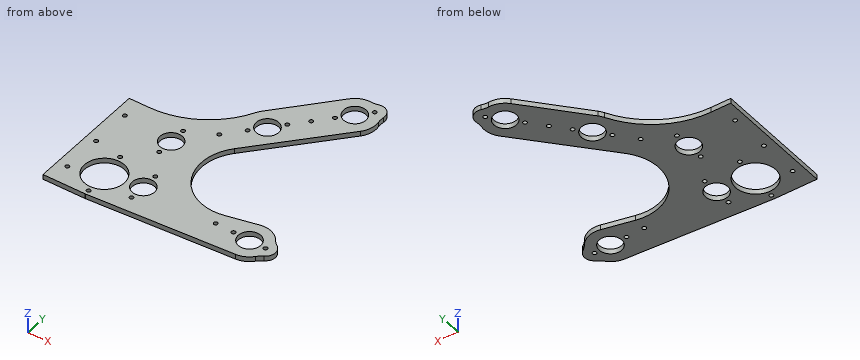
Autodesk Inventor part; units mm, degrees
ref_plane "YZ Plane" through (0, 0, 0) normal (1, 0, 0) x (0, 1, 0)
ref_plane "XZ Plane" through (0, 0, 0) normal (0, 1, 0) x (-1, 0, 0)
ref_plane "XY Plane" through (0, 0, 0) normal (0, 0, 1) x (1, 0, 0)
sketch "Sketch1" plane through (0, 0, 0) normal (0, 0, 1) x (1, 0, 0)
  line L0 (0, 0) -> (704.681, 0) construction
  line L1 (704.681, 0) -> (704.681, 101.6) construction
  line L2 (704.681, 101.6) -> (0, 101.6) construction
  circle A0 centre (304.8, 38.1) radius 38.1 construction
  circle A1 centre (212.725, 197.5786) radius 38.1 construction
  circle A2 centre (274.2046, 266.7) radius 38.1 construction
  circle A3 centre (499.5893, 180.5177) radius 203.2 construction
  line L3 (78.3329, 304.8) -> (550.894, 304.8) construction
  circle A4 centre (247.764, 111.4893) radius 57.15 construction
  circle A5 centre (258.7625, 117.8393) radius 53.975 construction
  line L4 (212.725, 197.5786) -> (304.8, 38.1) construction
  line L5 (258.7625, 117.8393) -> (247.764, 111.4893) construction
  line L6 (274.2046, 266.7) -> (212.725, 197.5786) construction
  dimension "d0" = 101.6
  dimension "d2" = 76.2
  dimension "d3" = 76.2
  dimension "d4" = 76.2
  dimension "d8" = 406.4
  dimension "d9" = 304.8
  dimension "d11" = 304.8
  dimension "d13" = 114.3
  dimension "d14" = 107.95
  dimension "d15" = 12.7
  dimension "d16" = 92.5068
  dimension "d17" = 60
sketch "Sketch4" plane through (0, 0, 0) normal (0, 0, 1) x (1, 0, 0)
  circle A0 centre (274.2046, 266.7) radius 38.1 construction
  circle A1 centre (212.725, 197.5786) radius 38.1 construction
  circle A2 centre (247.764, 111.4893) radius 57.15 construction
  circle A3 centre (304.8, 38.1) radius 38.1 construction
  circle A4 centre (274.2046, 266.7) radius 14.2875
  circle A5 centre (212.725, 197.5786) radius 14.2875
  circle A6 centre (304.8, 38.1) radius 14.2875
  circle A7 centre (145.2547, 121.0056) radius 39.6875 construction
  circle A8 centre (165.2583, 44.1925) radius 39.6875 construction
  circle A9 centre (145.2547, 121.0056) radius 14.2875
  circle A10 centre (165.2583, 44.1925) radius 14.2875
  line L0 (304.8, 38.1) -> (165.2583, 44.1925) construction
  line L1 (145.2547, 121.0056) -> (212.725, 197.5786) construction
  circle A11 centre (165.2583, 44.1925) radius 23.876 construction
  circle A12 centre (145.2547, 121.0056) radius 23.876 construction
  line L2 (128.9029, 138.4033) -> (202.94, 207.9895) construction
  line L3 (164.5725, 106.974) -> (224.2849, 189.182) construction
  line L4 (165.8568, 20.324) -> (305.1581, 23.817) construction
  line L5 (306.4016, 52.2974) -> (167.9348, 67.918) construction
  circle A13 centre (120.0426, 37.9792) radius 5.9531 construction
  circle A14 centre (120.0426, 37.9792) radius 25.4
  circle A15 centre (117.2754, 69.6084) radius 6.35 construction
  circle A16 centre (122.8098, 6.35) radius 6.35 construction
  line L6 (117.2754, 69.6084) -> (122.8098, 6.35) construction
  line L7 (0, 0) -> (304.8, 0) construction
  line L8 (69.2426, 0) -> (94.6426, 0) construction
  line L9 (94.6426, 0) -> (94.6426, 152.4) construction
  line L10 (94.6426, 152.4) -> (69.2426, 152.4)
  line L11 (69.2426, 152.4) -> (69.2426, 0)
  line L12 (81.9426, 127) -> (81.9426, 25.4) construction
  line L13 (283.8015, 39.0168) -> (325.7985, 37.1832) construction
  line L14 (260.2358, 250.9949) -> (288.1734, 282.4051) construction
  line L15 (145.2547, 99.9871) -> (145.2547, 142.0241) construction
  line L16 (165.2583, 23.174) -> (165.2583, 65.211) construction
  line L17 (226.6204, 213.3487) -> (198.8296, 181.8085) construction
  circle A17 centre (304.8, 38.1) radius 26.9875 construction
  circle A18 centre (325.7985, 37.1832) radius 12.7 construction
  circle A19 centre (288.1734, 282.4051) radius 12.7 construction
  line L18 (274.2046, 266.7) -> (212.725, 197.5786) construction
  circle A20 centre (274.2046, 266.7) radius 26.9875 construction
  circle A21 centre (212.725, 197.5786) radius 26.9875 construction
  arc A22 (94.6426, 152.4) -> (188.7085, 209.8884) centre (94.6426, 258.1022) ccw
  line L19 (254.0394, 284.6358) -> (192.5598, 215.5143)
  arc A23 (280.9291, 292.8363) -> (254.0394, 284.6358) centre (274.2046, 266.7) ccw
  arc A24 (299.3783, 276.4268) -> (280.9291, 292.8363) centre (288.1734, 282.4051) ccw
  line L20 (205.2733, 149.7079) -> (294.2696, 248.6523)
  arc A25 (205.2733, 149.7079) -> (260.3346, 55.7389) centre (247.764, 111.4893) ccw
  line L21 (260.3346, 55.7389) -> (298.8639, 64.4266)
  arc A26 (294.2696, 248.6523) -> (299.3783, 276.4268) centre (274.2046, 266.7) ccw
  arc A27 (192.5598, 215.5143) -> (188.7085, 209.8884) centre (212.725, 197.5786) ccw
  arc A28 (329.3139, 49.387) -> (298.8639, 64.4266) centre (304.8, 38.1) ccw
  arc A29 (328.2369, 24.7195) -> (329.3139, 49.387) centre (325.7985, 37.1832) ccw
  line L22 (306.4392, 11.1623) -> (123.1955, 0.0117)
  line L23 (69.2426, 0) -> (122.8098, 0)
  arc A30 (122.8098, 0) -> (123.1955, 0.0117) centre (122.8098, 6.35) ccw
  arc A31 (306.4392, 11.1623) -> (328.2369, 24.7195) centre (304.8, 38.1) ccw
  circle A32 centre (120.0426, 37.9792) radius 9.525 construction
  circle A33 centre (120.0426, 37.9792) radius 17.4625 construction
  circle A34 centre (260.3923, 40.0389) radius 6.35 construction
  point P0 (81.9426, 76.2)
  point P1 (94.6426, 76.2)
  point P2 (81.9426, 152.4)
  point P3 (243.4648, 232.1393)
  point P4 (118.5207, 55.3752)
  point P5 (178.9898, 159.2921)
  point P6 (104.2162, 45.3592)
  point P7 (105.7382, 27.9631)
  point P8 (121.5646, 20.5831)
  point P9 (135.869, 30.5992)
  point P10 (134.3471, 47.9953)
  dimension "d81" = 34.925
  dimension "d63" = 28.575
  dimension "d64" = 79.375
  dimension "d65" = 47.752
  dimension "d66" = 139.6746
  dimension "d67" = 102.0572
  dimension "d68" = 11.9062
  dimension "d69" = 50.8
  dimension "d70" = 12.7
  dimension "d71" = 2.5
  dimension "d72" = 85
  dimension "d73" = 25.4
  dimension "d74" = 152.4
  dimension "d75" = 101.6
  dimension "d76" = 42.037
  dimension "d77" = 12.7
  dimension "d79" = 25.4
  dimension "d80" = 19.05
  dimension "d92" = 12.7
  dimension "d95" = 360
extrude "Extrusion2" add sketch "Sketch4" along normal blind 6.35
hole "Hole2" at (117.2754, 69.6084, 0) at (122.8098, 6.35, 0) at (81.9426, 127, 0) at (81.9426, 76.2, 0) at (81.9426, 25.4, 0) at (283.8015, 39.0168, 0) at (325.7985, 37.1832, 0) at (260.2358, 250.9949, 0) at (288.1734, 282.4051, 0) at (145.2547, 142.0241, 0) at (145.2547, 99.9871, 0) at (165.2583, 65.211, 0) at (165.2583, 23.174, 0) at (198.8296, 181.8085, 0) at (226.6204, 213.3487, 0) at (243.4648, 232.1393, 0) at (118.5207, 55.3752, 0) at (260.3923, 40.0389, 0) at (178.9898, 159.2921, 0) at (134.3471, 47.9953, 0) at (135.869, 30.5992, 0) at (121.5646, 20.5831, 0) at (105.7382, 27.9631, 0) at (104.2162, 45.3592, 0) direction (0, 0, 1) diameter 5.1054 end through all
fillet "Fillet2" radius 25.4 4 edges at (299.3783, 276.4268, 3.175) (280.9291, 292.8363, 3.175) (329.3139, 49.387, 3.175) (328.2369, 24.7195, 3.175)
properties part number "GP8-002" material "Polycarbonate, Smoke"
Design review of the part built by this model. Coordinates are the model's own, in mm. Coordinates: 2 decimals unless noted, no trailing zeros. Loops run counter-clockwise (first coordinate to the right, second up) from the corner with the lowest first, then second, coordinate; pieces in that order, holes last. Notation, with made-up numbers: (-36, 37.5) - (10, 37.5) arc R6 cw to (10, 46.5) - close; hole circle Ø7 at (5, 64.5). An arc over 180 degrees is marked (long way). Use CSV: the item, a comma, the result in double quotes. Start each with the question number.
1. Add section A-A on x = 137. Give the boundary of the cut face in (y, z), plus the area to 3 significant figures.
2. Clearance check with flat-ended pins moving along their axes: pin 1 (23 mm diameter, centred on x = 145.25, y = 121.01, fed in from -Z); pin 2 (8 mm diameter, centred on x = 145.25, y = 99.99, fed in from +Z); pin 3 (3 mm diameter, centred on x = 269.5, z = 2, fed in from -Y); pin 4 (3 mm diameter, centred on x = 88, z = 4.5, fed in from +Y). State where each tip first meets the part, or that it passes through.
3. To check wall thickness, follow probe 1 along X at (y, z) = (48.5, 4.25); probe 2 along Y at (x, z) = (118, 1); probe 3 along Y at (x, z) = (122, 1.5). State the ranges of each line that lie inside material, in increasing order.
4. Add section D-D on x = 215. Give the boundary of the cut face in (y, z).
5. Add section B-B on x = 98.5. Give the boundary of the cut face in (y, z), plus the area to 3 significant figures.
6. Add section C-C on z = 3.25. Count the separate pieces of the cut face and the enclosed holes in it, plus the area to 3 significant figures.
Resolved:
1,outline,"(0.85, 0) - (19.07, 0) - (19.07, 6.35) - (0.85, 6.35) - close; (56.89, 0) - (109.34, 0) - (109.34, 6.35) - (56.89, 6.35) - close; (132.67, 0) - (161.26, 0) - (161.26, 6.35) - (132.67, 6.35) - close"
1,area,"630 mm2"
2,pin 1,"through"
2,pin 2,"z = 6.35"
2,pin 3,"y = 8.82"
2,pin 4,"y = 152.4"
3,probe 1,"69.24 to 96.92, 143.16 to 151.64, 178.88 to 295, 314.6 to 331.83"
3,probe 2,"0 to 12.66, 63.3 to 67.16, 72.06 to 155.01"
3,probe 3,"0 to 3.93, 8.77 to 12.65, 63.3 to 156"
4,outline,"(5.6, 0) - (64.66, 0) - (64.66, 6.35) - (5.6, 6.35) - close; (160.52, 0) - (183.47, 0) - (183.47, 6.35) - (160.52, 6.35) - close; (211.68, 0) - (240.74, 0) - (240.74, 6.35) - (211.68, 6.35) - close"
5,outline,"(0, 0) - (24.52, 0) - (24.52, 6.35) - (0, 6.35) - close; (51.44, 0) - (152.47, 0) - (152.47, 6.35) - (51.44, 6.35) - close"
5,area,"797 mm2"
6,separate pieces,"1"
6,enclosed holes,"24"
6,area,"30,100 mm2"
